```python
from build123d import *

# Parameters (mm, degrees)
F3_DEPTH = 25.4


with BuildPart() as f1:
    # F0 (on Front) → F1 (revolve)
    with BuildSketch(Plane.XZ):
        Polygon((-123.19, 0), (0, 0), (0, 5.08), (-118.11, 5.08), (-118.11, 43.18), (-146.05, 43.18), (-146.05, 0), (-140.97, 0), (-140.97, 38.1), (-123.19, 38.1), align=None)
    revolve(axis=Axis((0, 0, 2.54), (0, 0, -1)))

    # F2 (on face) → F3 (cut)
    with BuildSketch(Plane.XY.offset(5.08)):
        with BuildLine():
            Line((2.54, 12.264205), (2.54, 101.426891))
            Line((2.54, 101.426891), (2.54, 101.6))
            ThreePointArc((2.54, 101.6), (0, 104.05492), (-2.54, 101.6))
            Line((-2.54, 101.6), (-2.54, 101.426891))
            Line((-2.54, 101.426891), (-2.54, 12.264205))
            ThreePointArc((-2.54, 12.264205), (-4.107984, 9.917551), (-6.876051, 10.468154))
            Line((-6.876051, 10.468154), (-69.923591, 73.515693))
            Line((-69.923591, 73.515693), (-70.045998, 73.6381))
            ThreePointArc((-70.045998, 73.6381), (-73.577939, 73.577939), (-73.6381, 70.045998))
            Line((-73.6381, 70.045998), (-73.515693, 69.923591))
            Line((-73.515693, 69.923591), (-10.468154, 6.876051))
            ThreePointArc((-10.468154, 6.876051), (-9.917551, 4.107984), (-12.264205, 2.54))
            Line((-12.264205, 2.54), (-101.426891, 2.54))
            Line((-101.426891, 2.54), (-101.6, 2.54))
            ThreePointArc((-101.6, 2.54), (-104.05492, 0), (-101.6, -2.54))
            Line((-101.6, -2.54), (-101.426891, -2.54))
            Line((-101.426891, -2.54), (-12.264205, -2.54))
            ThreePointArc((-12.264205, -2.54), (-9.917551, -4.107984), (-10.468154, -6.876051))
            Line((-10.468154, -6.876051), (-73.515693, -69.923591))
            Line((-73.515693, -69.923591), (-73.6381, -70.045998))
            ThreePointArc((-73.6381, -70.045998), (-73.577939, -73.577939), (-70.045998, -73.6381))
            Line((-70.045998, -73.6381), (-69.923591, -73.515693))
            Line((-69.923591, -73.515693), (-6.876051, -10.468154))
            ThreePointArc((-6.876051, -10.468154), (-4.107984, -9.917551), (-2.54, -12.264205))
            Line((-2.54, -12.264205), (-2.54, -101.426891))
            Line((-2.54, -101.426891), (-2.54, -101.6))
            ThreePointArc((-2.54, -101.6), (0, -104.05492), (2.54, -101.6))
            Line((2.54, -101.6), (2.54, -101.426891))
            Line((2.54, -101.426891), (2.54, -12.264205))
            ThreePointArc((2.54, -12.264205), (4.107984, -9.917551), (6.876051, -10.468154))
            Line((6.876051, -10.468154), (69.923591, -73.515693))
            Line((69.923591, -73.515693), (70.045998, -73.6381))
            ThreePointArc((70.045998, -73.6381), (73.577939, -73.577939), (73.6381, -70.045998))
            Line((73.6381, -70.045998), (73.515693, -69.923591))
            Line((73.515693, -69.923591), (10.468154, -6.876051))
            ThreePointArc((10.468154, -6.876051), (9.917551, -4.107984), (12.264205, -2.54))
            Line((12.264205, -2.54), (101.426891, -2.54))
            Line((101.426891, -2.54), (101.6, -2.54))
            ThreePointArc((101.6, -2.54), (104.05492, 0), (101.6, 2.54))
            Line((101.6, 2.54), (101.426891, 2.54))
            Line((101.426891, 2.54), (12.264205, 2.54))
            ThreePointArc((12.264205, 2.54), (9.917551, 4.107984), (10.468154, 6.876051))
            Line((10.468154, 6.876051), (73.515693, 69.923591))
            Line((73.515693, 69.923591), (73.6381, 70.045998))
            ThreePointArc((73.6381, 70.045998), (73.577939, 73.577939), (70.045998, 73.6381))
            Line((70.045998, 73.6381), (69.923591, 73.515693))
            Line((69.923591, 73.515693), (6.876051, 10.468154))
            ThreePointArc((6.876051, 10.468154), (4.107984, 9.917551), (2.54, 12.264205))
        make_face()
    extrude(amount=-F3_DEPTH, mode=Mode.SUBTRACT)


solid = f1.part
```
Input: part model. Units: mm. Frame: model coordinates. A direction names the side the tool comes from. Coordinates: 2 decimals unless noted, no trailing zeros. Write each loop counter-clockwise with the first axis right and the second up, starting at its lowest first coordinate (ties: lowest second). Pieces come first, ordered by that corner, then holes. Notation, with made-up numbers: (35, 21) - (71, 21) arc R32 ccw to (71, 48) - close; hole circle Ø6 at (24, 82). An arc over 180 degrees is marked (long way). Put each result on its own line as item: value. Start each with the question number.
1) Mould query, pull axis X, two halves, no side actions, for faces 1 (the face through (118.3, 0.7, 43.18)), 2 (the face through (-134.46, 42.34, 19.32)), 3 (the face through (26.71, -120.26, 18.78)), 4 (the face through (-139.306, 43.869, 21.288)). Classes: pulls with the +X half, pulls with the -X half, needs draft (parallel to the pull), parting line crosses it, or undercut.
2) Contact query for flat-ended pins moving along their axis: pin 1 (1.5 mm diameter, centred on y = 37.5, z = 3, fed in from -X); pin 2 (2 mm diameter, centred on y = 107, z = 9.5, fed in from +X); pin 3 (2.5 mm diameter, centred on x = 50.5, z = 3, fed in from -Y). Output: stop coordinate, or through.
3) Cut plane B-B (x = 31). Return the cut outline in (y, z).
4) Cut plane A-A (y = -57.5). Return the cut outline in (x, z), plus the area to 3 significant figures.
5) Ray query, L1, parallel to Y at x = 0, z = 28; L2, parallel to X at y = 3.5, z = 6; L3, parallel to X at y = -59.5, z = 32. Return the intervals inside material, ascending.
6) Reachability of faces 5 (the face through (-109.104, -45.237, 24.397)), 6 (the face through (1, -125, 38.1)), 7 (the face through (-26, -53, 0)) from +Z, -Z, +X, -X, +Y, -Y: full face, straight path, thin tool, end or side. Return the list, or none.
7) Cut plane C-C (z = 28). Return the cut outline in (x, y).
Resolved:
1. face 1: needs draft
1. face 2: undercut
1. face 3: undercut
1. face 4: parting line crosses it
2. pin 1: stops at x = -141.35
2. pin 2: stops at x = 100.47
2. pin 3: stops at y = -137.5
3. outline: (-142.72, 0) - (-137.52, 0) - (-137.52, 38.1) - (-119.23, 38.1) - (-119.23, 0) - (-34.59, 0) - (-34.59, 5.08) - (-113.97, 5.08) - (-113.97, 43.18) - (-142.72, 43.18) - close; (-27.41, 0) - (-2.54, 0) - (-2.54, 5.08) - (-27.41, 5.08) - close; (2.54, 0) - (27.41, 0) - (27.41, 5.08) - (2.54, 5.08) - close; (34.59, 0) - (119.23, 0) - (119.23, 38.1) - (137.52, 38.1) - (137.52, 0) - (142.72, 0) - (142.72, 43.18) - (113.97, 43.18) - (113.97, 5.08) - (34.59, 5.08) - close
4. outline: (-134.25, 0) - (-128.71, 0) - (-128.71, 38.1) - (-108.95, 38.1) - (-108.95, 0) - (-61.09, 0) - (-61.09, 5.08) - (-103.17, 5.08) - (-103.17, 43.18) - (-134.25, 43.18) - close; (-53.91, 0) - (-2.54, 0) - (-2.54, 5.08) - (-53.91, 5.08) - close; (2.54, 0) - (53.91, 0) - (53.91, 5.08) - (2.54, 5.08) - close; (61.09, 0) - (108.95, 0) - (108.95, 38.1) - (128.71, 38.1) - (128.71, 0) - (134.25, 0) - (134.25, 43.18) - (103.17, 43.18) - (103.17, 5.08) - (61.09, 5.08) - close
4. area: 2,130 mm2
5. L1: y = -146.05 to -140.97, -123.19 to -118.11, 118.11 to 123.19, 140.97 to 146.05
5. L2: x = -146.01 to -140.93, -123.14 to -118.06, 118.06 to 123.14, 140.93 to 146.01
5. L3: x = -133.38 to -127.8, -107.87 to -102.03, 102.03 to 107.87, 127.8 to 133.38
6. face 5: +Z
6. face 6: -Z
6. face 7: -Z, +X, -X, +Y, -Y
7. outline: circle Ø292.1 at (0, 0); circle Ø246.38 at (0, 0); hole circle Ø281.94 at (0, 0); hole circle Ø236.22 at (0, 0)
